Check sheet for the modelled part. Datum: model origin and axes. Units: mm. A direction names the side the tool comes from. Round coordinates to 2 decimals unless told otherwise and drop trailing zeros. Write each loop counter-clockwise with the first axis right and the second up, starting at its lowest first coordinate (ties: lowest second). Pieces come first, ordered by that corner, then holes. Notation, with made-up numbers: (-5.75, -37.5) -> (16.25, -37.5) arc R31 ccw to (16.25, -5.5) -> close; hole circle Ø9 at (-3, -23). An arc over 180 degrees is marked (long way). One line per item, written item: value.
from build123d import *

# Parameters (mm, degrees)
SKETCH1_R                 = 77.5
SKETCH1_R_2               = 22
BOSS_EXTRUDE1_DEPTH       = 4
BOSS_EXTRUDE2_START       = -5
SKETCH1_4_R               = 25
BOSS_EXTRUDE2_DEPTH       = 5
BOSS_EXTRUDE5_START       = -50
SKETCH1_7_R               = 77.5
BOSS_EXTRUDE5_DEPTH       = 50
BOSS_EXTRUDE11_DEPTH      = 35
BOSS_EXTRUDE11_DEPTH_BACK = 35
FILLET6_R                 = 1
SKETCH1_8_R               = 77.5
BOSS_EXTRUDE12_DEPTH      = 5
SKETCH9_W                 = 28.884835104
SKETCH9_H                 = 19.109753223
BOSS_EXTRUDE15_DEPTH      = 5
SKETCH10_W                = 6.135894163
SKETCH10_H                = 2.546187374
SKETCH10_W_2              = 6.094153386
CUT_EXTRUDE1_DEPTH        = 19.109753223
SKETCH9_9_W               = 4.209300424
SKETCH9_9_H               = 19.109753223
BOSS_EXTRUDE16_DEPTH      = 10


with BuildPart() as part:
    # Sketch1 → Boss-Extrude1 (new body)
    with BuildSketch(Plane(origin=(-55.630480005, 66.15900607, 0), x_dir=(0.499999999999998, 0.8660254037844398, 0), z_dir=(0, 0, 1))):
        with BuildLine():
            Line((-189.316298544, 16.630324375), (-62.719050458, 92.734061587))
            ThreePointArc((-62.719050458, 92.734061587), (-39.919544136, 96.109788868), (-21.454102902, 82.317018907))
            Line((-21.454102902, 82.317018907), (42.273246416, -25.216830667))
            ThreePointArc((42.273246416, -25.216830667), (45.552356682, -47.854466687), (31.921457021, -66.223290906))
            Line((31.921457021, -66.223290906), (-94.675791065, -142.327028118))
            ThreePointArc((-94.675791065, -142.327028118), (-117.475297387, -145.7027554), (-135.940738621, -131.909985438))
            Line((-135.940738621, -131.909985438), (-199.668087939, -24.376135865))
            ThreePointArc((-199.668087939, -24.376135865), (-202.947198205, -1.738499844), (-189.316298544, 16.630324375))
        make_face()
        with Locations(Location((-62.487009575, -8.6321901, 0), (0, 0, 300))):
            Circle(SKETCH1_R, mode=Mode.SUBTRACT)
        with Locations(Location((-108.711062401, -106.957491085, 0), (0, 0, 300))):
            Circle(SKETCH1_R_2, mode=Mode.SUBTRACT)
    extrude(amount=BOSS_EXTRUDE1_DEPTH)

    # Sketch1_4 → Boss-Extrude2 (add)
    with BuildSketch(Plane(origin=(-55.630480005, 66.15900607, 0), x_dir=(0.499999999999998, 0.8660254037844398, 0), z_dir=(0, 0, 1)).offset(BOSS_EXTRUDE2_START)):
        with BuildLine():
            Line((-189.316298544, 16.630324375), (-62.719050458, 92.734061587))
            ThreePointArc((-62.719050458, 92.734061587), (-39.919544136, 96.109788868), (-21.454102902, 82.317018907))
            Line((-21.454102902, 82.317018907), (42.273246416, -25.216830667))
            ThreePointArc((42.273246416, -25.216830667), (45.552356682, -47.854466687), (31.921457021, -66.223290906))
            Line((31.921457021, -66.223290906), (-94.675791065, -142.327028118))
            ThreePointArc((-94.675791065, -142.327028118), (-117.475297387, -145.7027554), (-135.940738621, -131.909985438))
            Line((-135.940738621, -131.909985438), (-199.668087939, -24.376135865))
            ThreePointArc((-199.668087939, -24.376135865), (-202.947198205, -1.738499844), (-189.316298544, 16.630324375))
        make_face()
        with Locations(Location((-108.711062401, -106.957491085, 0), (0, 0, 300))):
            Circle(SKETCH1_4_R, mode=Mode.SUBTRACT)
    extrude(amount=BOSS_EXTRUDE2_DEPTH)

    # Sketch1_7 → Boss-Extrude5 (add)
    with BuildSketch(Plane(origin=(-55.630480005, 66.15900607, 0), x_dir=(0.499999999999998, 0.8660254037844398, 0), z_dir=(0, 0, 1)).offset(BOSS_EXTRUDE5_START)):
        with Locations(Location((-62.487009575, -8.6321901, 0), (0, 0, 300))):
            Circle(SKETCH1_7_R)
        Polygon((-84.859101961, 59.5935777), (-112.245619562, 43.13021558), (-129.776834206, 16.41467419), (-133.980473825, -15.261705851), (-124.023956041, -45.625028993), (-101.879291307, -68.661466704), (-71.932502062, -79.808369973), (-40.114917188, -76.8579579), (-12.728399587, -60.39459578), (4.802815056, -33.679054391), (9.006454676, -2.002674349), (-0.950063109, 28.360648792), (-23.094727842, 51.397086504), (-53.041517088, 62.543989773), align=None, mode=Mode.SUBTRACT)
    extrude(amount=BOSS_EXTRUDE5_DEPTH)

    # Sketch8 → Boss-Extrude11 (add, two sides: drawn at the far end of the back side and taken through both)
    with BuildSketch(Plane(origin=(-78.84892316, -0.897416974, 0), x_dir=(0, 0, 1), z_dir=(0.9999352373159692, 0.01138073696455021, 0)).offset(-BOSS_EXTRUDE11_DEPTH_BACK)):
        Polygon((-23.295016777, 86.56703586), (-18.615876211, 86.56703586), (-18.615875095, 65.56703586), (-41.615875095, 65.56703586), (-41.615876211, 86.56703586), (-36.936735645, 86.56703586), (-39.315876073, 83.96703586), (-39.315875265, 68.76703586), (-20.915875265, 68.76703586), (-20.915876073, 83.96703586), align=None)
    extrude(amount=BOSS_EXTRUDE11_DEPTH + BOSS_EXTRUDE11_DEPTH_BACK)

    # Fillet6
    fillet6_edges = [part.edges().sort_by_distance(p)[0] for p in [
        (-77.863726496, -87.45884652, -23.295016777),
        (-42.86599319, -87.060520726, -20.955446494),
        (-77.863726496, -87.45884652, -18.615876211),
        (-77.863726496, -87.45884652, -41.615876211),
        (-42.86599319, -87.060520726, -39.276305928),
        (-77.863726496, -87.45884652, -36.936735645),
        (-77.893316412, -84.859014903, -39.315876073),
        (-77.893316412, -84.859014903, -20.915876073),
        (-112.861459802, -87.857172313, -20.955446494),
        (-112.861459802, -87.857172313, -39.276305928),
    ]]
    fillet(fillet6_edges, radius=FILLET6_R)

    # Sketch1_8 → Boss-Extrude12 (add)
    # profile 1 of 2: a face of its own
    with BuildSketch(Plane(origin=(-55.630480005, 66.15900607, 0), x_dir=(0.499999999999998, 0.8660254037844398, 0), z_dir=(0, 0, 1))):
        with Locations(Location((-62.487009575, -8.6321901, 0), (0, 0, 300))):
            Circle(SKETCH1_8_R)
        Polygon((-53.041517088, 62.543989773), (-84.859101961, 59.5935777), (-112.245619562, 43.13021558), (-129.776834206, 16.41467419), (-133.980473825, -15.261705851), (-124.023956041, -45.625028993), (-101.879291307, -68.661466704), (-71.932502062, -79.808369973), (-40.114917188, -76.8579579), (-12.728399587, -60.39459578), (4.802815056, -33.679054391), (9.006454676, -2.002674349), (-0.950063109, 28.360648792), (-23.094727842, 51.397086504), align=None, mode=Mode.SUBTRACT)
    # profile 2 of 2: a face of its own
    with BuildSketch(Plane(origin=(-55.630480005, 66.15900607, 0), x_dir=(0.499999999999998, 0.8660254037844398, 0), z_dir=(0, 0, 1))):
        Polygon((-23.094727842, 51.397086504), (-53.041517088, 62.543989773), (-84.859101961, 59.5935777), (-112.245619562, 43.13021558), (-129.776834206, 16.41467419), (-133.980473825, -15.261705851), (-124.023956041, -45.625028993), (-101.879291307, -68.661466704), (-71.932502062, -79.808369973), (-40.114917188, -76.8579579), (-12.728399587, -60.39459578), (4.802815056, -33.679054391), (9.006454676, -2.002674349), (-0.950063109, 28.360648792), align=None)
    extrude(amount=BOSS_EXTRUDE12_DEPTH)

    # Sketch9 → Boss-Extrude15 (add)
    with BuildSketch(Plane(origin=(0, 0, -5), x_dir=(-1, 0, 0), z_dir=(0, 0, -1))):
        with Locations((147.381235027, -73.319519351)):
            Rectangle(SKETCH9_W, SKETCH9_H)
    extrude(amount=BOSS_EXTRUDE15_DEPTH)

    # Sketch10 → Cut-Extrude1 (cut)
    with BuildSketch(Plane.XZ.offset(82.874395962)):
        with Locations((-141.22663524, -7.28335185)):
            Rectangle(SKETCH10_W, SKETCH10_H)
        with Locations((-154.687790802, -7.28335185)):
            Rectangle(SKETCH10_W_2, SKETCH10_H)
    extrude(amount=-CUT_EXTRUDE1_DEPTH, mode=Mode.SUBTRACT)

    # Sketch9_9 → Boss-Extrude16 (add)
    with BuildSketch(Plane(origin=(0, 0, -5), x_dir=(-1, 0, 0), z_dir=(0, 0, -1))):
        with Locations((130.834167263, -73.319519351)):
            Rectangle(SKETCH9_9_W, SKETCH9_9_H)
    extrude(amount=BOSS_EXTRUDE16_DEPTH)


solid = part.part
Item 1: Mould release check, pull along Z, two halves, no side actions. Record for faces 1 (the flat face through (-62.836, -60.285, -27.815)), 2 (the flat face through (-155, -73, -8.556)), 3 (the flat face through (-78, -76, -41.616)): pulls with the +Z half, pulls with the -Z half, needs draft (parallel to the pull), parting line crosses it, or undercut.
Answer:
face 1: needs draft
face 2: undercut
face 3: pulls with the -Z half
Item 2: Tool access check on faces 4 (the flat face through (-141, -82.874, -9)), 5 (the flat face through (-36.55, 63.08, -27.82)), 6 (the flat face through (-128.73, -73, -10)). Record the directions out of +Z, -Z, +X, -X, +Y, -Y that give a thin tool (end or side, any length) a straight path to the whole face; none if there is none.
Answer:
face 4: -Z, +X, -X, -Y
face 5: -Z
face 6: -Z, -Y
Item 3: Thickness scan on line 1 (Y direction, x = -47, z = -38.5); line 2 (Y direction, x = -45, z = -41.5); line 3 (Z direction, x = -110.5, y = -106). Record the ranges inside material, lowest first.
Answer:
line 1: y = -86.81 to -85.4, -69.31 to -66.11, -62.68 to -56.31, 71.12 to 78.13
line 2: y = -86.55 to -66.08, -61.72 to -54.66, 69.58 to 77.18
line 3: z = -5 to 4
Item 4: Sectioned sample at B-B on y = -76. Count the separate pieces of the cut face and the enclosed holes in it, and give its area (3 significant figures).
Answer:
separate pieces: 4
enclosed holes: 2
area: 1,730 mm^2
Item 5: Sectioned sample at C-C on x = -17. Enter the section's corners in (y, z), and give its area (3 significant figures).
Answer:
outline: (-117.61, -5) -> (-106.46, -5) -> (-106.46, 0) -> (-103.46, 0) -> (-103.46, 4) -> (-117.61, 4) -> close; (-59.47, 0) -> (-56.47, 0) -> (-56.47, -5) -> (-38.24, -5) -> (-38.24, -50) -> (-24.13, -50) -> (-24.13, -5) -> (39.45, -5) -> (39.45, -50) -> (53.69, -50) -> (53.69, -5) -> (90.11, -5) -> (90.11, 4) -> (53.69, 4) -> (53.69, 5) -> (-38.24, 5) -> (-38.24, 4) -> (-59.47, 4) -> close
area: 2,810 mm^2
Item 6: Depth check by flat-ended pin: P1, Ø3.5, axis at x = -131, y = -73, coming from the -Z side; P2, Ø12, axis at x = -120, z = -8, coming from the +Y side; P3, Ø6.5, axis at x = -155, y = -71.5, coming from the +Z side. Enter the tip coordinate at first touch or a pass-through.
Answer:
P1: stops at z = -15
P2: stops at y = 89
P3: stops at z = 4
Item 7: Sectioned sample at A-A on z = -32. Enter the section's corners in (x, y), and give its area (3 significant figures).
Answer:
outline: (-113.1, -66.86) -> (-113.06, -70.06) -> (-82.5, -69.71) arc R77.5 ccw to (-74.54, -69.62) -> (-43.07, -69.26) -> (-43.1, -66.06) -> (-56.17, -66.21) arc R77.5 ccw (long way) to (-100.93, -66.72) -> close; hole (-149.67, 22.47) -> (-149.11, -9.48) -> (-134.73, -38.02) -> (-109.4, -57.5) -> (-78.13, -64.06) -> (-47.11, -56.4) -> (-22.48, -36.04) -> (-9.13, -7.01) -> (-9.69, 24.94) -> (-24.06, 53.48) -> (-49.39, 72.96) -> (-80.67, 79.52) -> (-111.69, 71.86) -> (-136.32, 51.5) -> close
area: 3,340 mm^2
Item 8: Sectioned sample at D-D on y = -44. Enter the section's corners in (x, z).
Answer:
outline: (-165.49, -5) -> (-137.11, -5) -> (-137.11, -50) -> (-126.96, -50) -> (-126.96, -5) -> (-32.11, -5) -> (-32.11, -50) -> (-21.69, -50) -> (-21.69, -5) -> (19.53, -5) -> (19.53, 4) -> (-21.69, 4) -> (-21.69, 5) -> (-137.11, 5) -> (-137.11, 4) -> (-165.49, 4) -> close
